Model file for the job. Use its own axes, mm. A direction names the side the tool comes from. Coordinates: 2 decimals unless noted, no trailing zeros. Loops run counter-clockwise (first coordinate to the right, second up) from the corner with the lowest first, then second, coordinate; pieces in that order, holes last. Notation, with made-up numbers: (62, -3.75) -> (87, -3.75) arc R32 cw to (87, 35.25) -> close; hole circle Ø8 at (74, -12.75). An arc over 180 degrees is marked (long way). Use one line per item in the form item = value.
```python
from build123d import *

# Parameters (mm, degrees)
SKETCH1_W           = 105
SKETCH1_H           = 4
SKETCH1_W_2         = 2
SKETCH1_H_2         = 9.75
BOSS_EXTRUDE1_DEPTH = 12.5
SKETCH2_W           = 8
SKETCH2_H           = 10
SKETCH2_R           = 1.55
BOSS_EXTRUDE2_DEPTH = 2
SKETCH4_W           = 8
SKETCH4_H           = 10
SKETCH4_R           = 1.55
BOSS_EXTRUDE3_DEPTH = 2
SKETCH5_W           = 101
SKETCH5_H           = 2
CUT_EXTRUDE1_DEPTH  = 4.75
SKETCH6_W           = 101
SKETCH6_H           = 2
CUT_EXTRUDE2_DEPTH  = 4.75
FILLET1_R           = 2


with BuildPart() as part:
    # Sketch1 → Boss-Extrude1 (new body, symmetric)
    with BuildSketch(Plane(origin=(0, 0, 0), x_dir=(0, 0, -1), z_dir=(1, 0, 0))):
        Rectangle(SKETCH1_W, SKETCH1_H)
        Polygon((-52.5, 63.25), (-52.5, 2), (-48.5, 2), (-48.5, 63.25), (-50.5, 63.25), align=None)
        Polygon((48.5, 63.25), (48.5, 2), (52.5, 2), (52.5, 63.25), (50.5, 63.25), align=None)
        with Locations((-49.5, 68.125)):
            Rectangle(SKETCH1_W_2, SKETCH1_H_2)
        with Locations((49.5, 68.125)):
            Rectangle(SKETCH1_W_2, SKETCH1_H_2)
    extrude(amount=BOSS_EXTRUDE1_DEPTH, both=True)

    # Sketch2 → Boss-Extrude2 (add)
    with BuildSketch(Plane.XY.offset(-48.5)):
        with Locations((-16.5, 16)):
            Rectangle(SKETCH2_W, SKETCH2_H)
        with Locations((-16.5, 16)):
            Circle(SKETCH2_R, mode=Mode.SUBTRACT)
        with Locations((-16.5, 44)):
            Rectangle(SKETCH2_W, SKETCH2_H)
        with Locations((-16.5, 44)):
            Circle(SKETCH2_R, mode=Mode.SUBTRACT)
        with Locations((16.5, 16)):
            Rectangle(SKETCH2_W, SKETCH2_H)
        with Locations((16.5, 16)):
            Circle(SKETCH2_R, mode=Mode.SUBTRACT)
        with Locations((16.5, 44)):
            Rectangle(SKETCH2_W, SKETCH2_H)
        with Locations((16.5, 44)):
            Circle(SKETCH2_R, mode=Mode.SUBTRACT)
    extrude(amount=-BOSS_EXTRUDE2_DEPTH)

    # Sketch4 → Boss-Extrude3 (add)
    with BuildSketch(Plane(origin=(0, 0, 48.5), x_dir=(-1, 0, 0), z_dir=(0, 0, -1))):
        with Locations((-16.5, 16)):
            Rectangle(SKETCH4_W, SKETCH4_H)
        with Locations((-16.5, 16)):
            Circle(SKETCH4_R, mode=Mode.SUBTRACT)
        with Locations((-16.5, 44)):
            Rectangle(SKETCH4_W, SKETCH4_H)
        with Locations((-16.5, 44)):
            Circle(SKETCH4_R, mode=Mode.SUBTRACT)
        with Locations((16.5, 16)):
            Rectangle(SKETCH4_W, SKETCH4_H)
        with Locations((16.5, 16)):
            Circle(SKETCH4_R, mode=Mode.SUBTRACT)
        with Locations((16.5, 44)):
            Rectangle(SKETCH4_W, SKETCH4_H)
        with Locations((16.5, 44)):
            Circle(SKETCH4_R, mode=Mode.SUBTRACT)
    extrude(amount=-BOSS_EXTRUDE3_DEPTH)

    # Sketch5 → Cut-Extrude1 (cut)
    with BuildSketch(Plane.ZY.offset(12.5)):
        Polygon((-50.5, 63.25), (-52.5, 63.25), (-52.5, -2), (-50.5, -2), (-50.5, 0), (-50.5, 11), (-50.5, 21), (-50.5, 39), (-50.5, 49), align=None)
        with Locations((0, -1)):
            Rectangle(SKETCH5_W, SKETCH5_H)
        Polygon((50.5, 0), (50.5, -2), (52.5, -2), (52.5, 63.25), (50.5, 63.25), (50.5, 49), (50.5, 39), (50.5, 21), (50.5, 11), align=None)
    extrude(amount=-CUT_EXTRUDE1_DEPTH, mode=Mode.SUBTRACT)

    # Sketch6 → Cut-Extrude2 (cut)
    with BuildSketch(Plane(origin=(12.5, 0, 0), x_dir=(0, 0, -1), z_dir=(1, 0, 0))):
        Polygon((-50.5, 0), (-50.5, 63.25), (-52.5, 63.25), (-52.5, -2), (-50.5, -2), align=None)
        with Locations((0, -1)):
            Rectangle(SKETCH6_W, SKETCH6_H)
        Polygon((50.5, 63.25), (50.5, 0), (50.5, -2), (52.5, -2), (52.5, 63.25), align=None)
    extrude(amount=-CUT_EXTRUDE2_DEPTH, mode=Mode.SUBTRACT)

    # Fillet1
    fillet1_edges = [part.edges().sort_by_distance(p)[0] for p in [
        (12.5, 21, 49.5),
        (12.5, 11, 49.5),
        (12.5, 49, 49.5),
        (12.5, 39, 49.5),
        (-12.5, 11, 49.5),
        (-12.5, 21, 49.5),
        (-12.5, 39, 49.5),
        (-12.5, 49, 49.5),
        (-12.5, 21, -49.5),
        (-12.5, 11, -49.5),
        (-12.5, 49, -49.5),
        (-12.5, 39, -49.5),
        (12.5, 11, -49.5),
        (12.5, 21, -49.5),
        (12.5, 39, -49.5),
        (12.5, 49, -49.5),
    ]]
    fillet(fillet1_edges, radius=FILLET1_R)


solid = part.part
```
Q1. Mould opens along Y. For faces 4 (the face through (0, 30, -52.5)), 5 (the face through (0, -2, 1)), 6 (the face through (-17.64, 17.05, -49.49)), 7 (the face through (-15.36, 17.05, 49.49)) say: released by +Y, released by -Y, zero draft, split by the parting line, or undercut.
Result:
face_4 = zero draft
face_5 = released by -Y
face_6 = undercut
face_7 = undercut
Q2. Band-saw the part on B-B, the plane x = 16.5. State how many separate pieces and enclosed holes the cut face has, and give its area (3 significant figures).
Result:
separate_pieces = 8
enclosed_holes = 0
area = 55.2 mm2
Q3. Wall check: line 1 along Y through (x, z) = (16.5, 49.8); line 2 along Z through (x, y) = (-2, 13); line 3 along Z through (x, y) = (-10.5, 11). Give the ranges that are in metal, low to high.
Result:
line_1 = 11 to 14.45, 17.55 to 21, 39 to 42.45, 45.55 to 49
line_2 = -52.5 to -48.5, 48.5 to 52.5
line_3 = -50.5 to -48.5, 48.5 to 50.5
Q4. Pin check, flat tips, straight feed: pin 1 Ø1 at (x, y) = (12.5, 16) entering from +Z; pin 2 Ø1 at (y, z) = (65.5, -49) entering from -X; pin 3 Ø0.6 at (y, z) = (31, -50) entering from +X; pin 4 Ø2.5 at (x, y) = (16.5, 16) entering from +Z (3 decimals). Stop position of each tip, or through.
Result:
pin_1 = 50.5
pin_2 = -12.5
pin_3 = 12.5
pin_4 = through
Q5. Band-saw the part on D-D, the plane z = 41.5. Write the cut outline in (x, y).
Result:
outline = (-12.5, 0) -> (-7.75, 0) -> (-7.75, -2) -> (7.75, -2) -> (7.75, 0) -> (12.5, 0) -> (12.5, 2) -> (-12.5, 2) -> close
Q6. Band-saw the part on A-A, the plane y = 64.5. Write the cut outline in (x, z), and give its area (3 significant figures).
Result:
outline = (-12.5, -50.5) -> (12.5, -50.5) -> (12.5, -48.5) -> (-12.5, -48.5) -> close; (-12.5, 48.5) -> (12.5, 48.5) -> (12.5, 50.5) -> (-12.5, 50.5) -> close
area = 100 mm2
Q7. Which spindle directions (+Z, -Z, +X, -X, +Y, -Y) get a long thin tool onto all of the face, cutting with end or side? Do faces 1 (the face through (0, 38, -48.5)), 2 (the face through (10, 0, 1)), 3 (the face through (-12.5, 1, 8)). Say none if no direction does.
Result:
face_1 = +X, -X, +Y
face_2 = +Z, -Z, +X, -Y
face_3 = +Z, -Z, -X, -Y
